Build history of the part. All positions in model axes, mm. Coordinates: 2 decimals unless noted, no trailing zeros. Order: outer loops, then holes, each group sorted by start corner. A loop starts at its lowest first (then second) coordinate and runs counter-clockwise, first axis right, second up. Notation, with made-up numbers: (46, 79) - (73, 79) arc R28 cw to (73, 113) - close; hole circle Ø10 at (3, 47). An arc over 180 degrees is marked (long way). Write each question's results on one line, items separated by ' | '.
from build123d import *

# Parameters (mm, degrees)
SKETCH1_R           = 2.5
BOSS_EXTRUDE1_DEPTH = 6
SKETCH2_R           = 0.25
BOSS_EXTRUDE2_DEPTH = 25


with BuildPart() as part:
    # Sketch1 → Boss-Extrude1 (new body)
    with BuildSketch(Plane.XY):
        Circle(SKETCH1_R)
    extrude(amount=BOSS_EXTRUDE1_DEPTH)

    # Sketch2 → Boss-Extrude2 (add)
    with BuildSketch(Plane.XY):
        with Locations((-1, 0)):
            Circle(SKETCH2_R)
        with Locations((1, 0)):
            Circle(SKETCH2_R)
    extrude(amount=-BOSS_EXTRUDE2_DEPTH)


solid = part.part
1. Band-saw the part on A-A on z = -22. Give the cut face in (x, y).
Solved:
outline: circle Ø0.5 at (-1, 0); circle Ø0.5 at (1, 0)
2. Probe line 1 (Z direction, x = 0.3, y = 1.9); line 2 (X direction, y = 0.15, z = -13); line 3 (Y direction, x = 1.1, z = -5.5). List the from-to ranges inside material, lowest first.
Solved:
line 1: z = 0 to 6 | line 2: x = -1.2 to -0.8, 0.8 to 1.2 | line 3: y = -0.23 to 0.23
3. Band-saw the part on C-C on y = -0.85. Give the cut face in (x, z), then the cut area to 3 significant figures.
Solved:
outline: (-2.35, 0) - (2.35, 0) - (2.35, 6) - (-2.35, 6) - close | area: 28.2 mm2
4. Two-plate mould, pull along Z, no slides. Class faces 1 (the face through (0, 0, 0)), 2 (the face through (0, 0, 6)), 3 (the face through (-0.54, -2.44, 2.96)): +Z half, -Z half, draft (parallel to the pull), parting line (faces both ways), or undercut.
Solved:
face 1: -Z half | face 2: +Z half | face 3: draft
5. Band-saw the part on B-B on x = 0. Give the cut face in (y, z).
Solved:
outline: (-2.5, 0) - (2.5, 0) - (2.5, 6) - (-2.5, 6) - close
6. Drop a flat-ended pin along its axis: pin 1 Ø1 at (y, z) = (2, -15.5) entering from -X (3 decimals). Give the stop position or say it passes through.
Solved:
pin 1: passes through
